from build123d import *

# Parameters (mm, degrees)
F0_W     = 152.907998
F0_H     = 55.118002
F1_DEPTH = 37.084
F2_T     = -2.54
F3_W     = 16.256001
F3_H     = 18.415
F4_DEPTH = 3.048
F6_DEPTH = 152.908
F7_W     = 10.667999
F7_H     = 9.906002
F8_DEPTH = 2.794


with BuildPart() as f1:
    # F0 (on Top) → F1 (new body)
    with BuildSketch(Plane.XY):
        Rectangle(F0_W, F0_H)
    extrude(amount=F1_DEPTH)

    # F2
    f2_openings = [f1.faces().sort_by_distance(p)[0] for p in [
        (0, 0, 37.084),
    ]]
    offset(amount=F2_T, openings=f2_openings)

    # F3 (on face) → F4 (cut)
    with BuildSketch(Plane.XZ.offset(27.559001)):
        with Locations((-24.765001, 9.2075)):
            Rectangle(F3_W, F3_H)
    extrude(amount=-F4_DEPTH, mode=Mode.SUBTRACT)

    # F5 (on face) → F6 (join)
    with BuildSketch(Plane.YZ.offset(76.453999)):
        Polygon((27.559001, 37.084), (0, 56.972686), (-27.559001, 37.084), align=None)
    extrude(amount=-F6_DEPTH)

    # F7 (on face) → F8 (cut)
    with BuildSketch(Plane.XZ.offset(27.559001)):
        with Locations((-65.658999, 22.098001)):
            Rectangle(F7_W, F7_H)
    extrude(amount=-F8_DEPTH, mode=Mode.SUBTRACT)


solid = f1.part
The listing builds one solid part. Answer for the finished solid, in the listing's coordinates (mm). A direction names the side the tool comes from. Coordinates: 2 decimals unless noted, no trailing zeros. Write each loop counter-clockwise with the first axis right and the second up, starting at its lowest first coordinate (ties: lowest second). Pieces come first, ordered by that corner, then holes. Notation, with made-up numbers: M -8,-13.75 L 27,-13.75 A18 cw 27,7.25 Z; hole C -36.5,59.25 d7. An arc over 180 degrees is marked long. Use one line per item in the form item = value.
Item 1: For faces 1 (the face through (73.914, 0, 20)), 2 (the face through (76.454, 0, 23)), 3 (the face through (-32.893, -26, 9)), determine the directions among +Z, -Z, +X, -X, +Y, -Y from which every point of the face is accessible in a straight line to the end or side of a thin tool.
Model answer:
face_1 = none
face_2 = +Z, -Z, +X, +Y, -Y
face_3 = -Z, -Y
Item 2: Find section C-C, the plane x = -54. Give the vertices of the cut face in (y, z), plus the area to 3 significant figures.
Model answer:
outline = M -27.56,0 L 27.56,0 L 27.56,37.08 L 0,56.97 L -27.56,37.08 Z; hole M -25.02,2.54 L 25.02,2.54 L 25.02,37.08 L -25.02,37.08 Z
area = 864 mm2
Item 3: The mould has two halves that part along Z. Classify faces 4 (the face through (-1, -25.019, 20)), 5 (the face through (-1, 27.559, 18)), 6 (the face through (-1, 0, 0)): released by +Z, released by -Z, zero draft, split by the parting line, or undercut.
Model answer:
face_4 = undercut
face_5 = zero draft
face_6 = released by -Z
Item 4: Find section B-B, the plane x = -29. Give the vertices of the cut face in (y, z) (3 decimals), plus the area to 3 significant figures.
Model answer:
outline = M -27.559,18.415 L -25.019,18.415 L -25.019,37.084 L 25.019,37.084 L 25.019,2.54 L -24.511,2.54 L -24.511,0 L 27.559,0 L 27.559,37.084 L 0,56.973 L -27.559,37.084 Z
area = 816 mm2
Item 5: Find the intervals of material crossed by probe 1 along X at (y, z) = (-9.5, 36.5); probe 2 along Y at (x, z) = (-7.5, 8); probe 3 along Z at (x, y) = (-67, -10), in increasing order.
Model answer:
probe_1 = -76.45 to -73.91, 73.91 to 76.45
probe_2 = -27.56 to -25.02, 25.02 to 27.56
probe_3 = 0 to 2.54, 37.08 to 49.76
Item 6: Find section A-A, the plane z = 29. Give the vertices of the cut face in (x, y).
Model answer:
outline = M -76.45,-27.56 L 76.45,-27.56 L 76.45,27.56 L -76.45,27.56 Z; hole M -73.91,-25.02 L 73.91,-25.02 L 73.91,25.02 L -73.91,25.02 Z
Item 7: Given P1, Ø2, axis at x = -68.5, y = -26, coming from the +Z side; P2, Ø2, axis at x = -24, y = -26, coming from the -Z side (3 decimals); P3, Ø3, axis at x = -27.5, z = 1, coming from the -Y side, each flat-ended and moving along its own axis, determine where each tip first touches the part or whether it passes through.
Model answer:
P1 = 38.93
P2 = 18.415
P3 = -24.51
